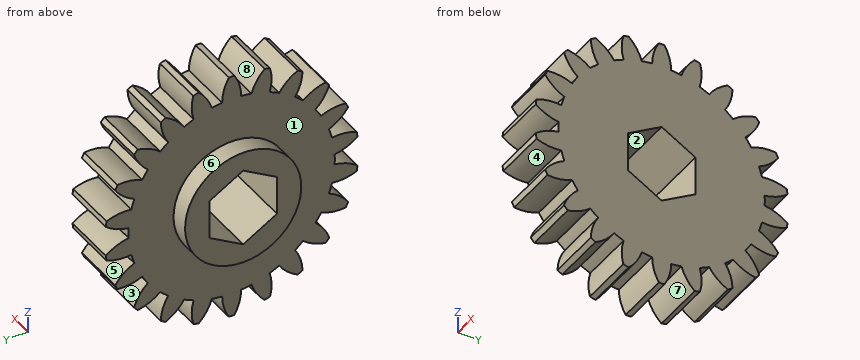
```python
from build123d import *

# Parameters (mm, degrees)
BASPROSKE_W         = 6.604
BASPROSKE_H         = 15.24
TOOTHCUT_DEPTH      = 23.541695056
TEETHCUTS_COUNT     = 22
TEETHCUTS_ANGLE     = 343.636363636
BORSKE_R            = 0.499999
BORE_DEPTH          = 50.8000508
SKETCH1_R           = 6.985
BOSS_EXTRUDE1_DEPTH = 2.286
CUT_EXTRUDE1_DEPTH  = 24.241702632


with BuildPart() as part:
    # BasProSke → Base-Revolve (revolve)
    with BuildSketch(Plane(origin=(0, 0, 0), x_dir=(1, 0, 0), z_dir=(0, 1, 0)), mode=Mode.PRIVATE) as base_revolve_sk:
        with Locations((3.302, 7.62)):
            Rectangle(BASPROSKE_W, BASPROSKE_H)
    revolve(base_revolve_sk.sketch.rotate(Axis((-10, 0, 0), (1, 0, 0)), 180), axis=Axis((-10, 0, 0), (1, 0, 0)))

    # TooCutSke → ToothCut (cut, through all)
    with BuildSketch(Plane(origin=(0, 0, 0), x_dir=(0, 0, -1), z_dir=(1, 0, 0))):
        with BuildLine():
            ThreePointArc((0.629474743, 12.379206137), (0, 12.3952), (-0.629474743, 12.379206137))
            ThreePointArc((-0.629474743, 12.379206137), (-1.05059125, 13.850443254), (-1.855031489, 15.152270303))
            ThreePointArc((-1.855031489, 15.152270303), (0, 15.2654), (1.855031489, 15.152270303))
            ThreePointArc((1.855031489, 15.152270303), (1.05059125, 13.850443254), (0.629474743, 12.379206137))
        make_face()
    toothcut = extrude(amount=TOOTHCUT_DEPTH, mode=Mode.SUBTRACT)

    # TeethCuts: ToothCut ×22 about axis
    teethcuts_axis = Axis((-10, 0, 0), (1, 0, 0))
    for i in range(1, TEETHCUTS_COUNT):
        add(toothcut.rotate(teethcuts_axis, i * TEETHCUTS_ANGLE / (TEETHCUTS_COUNT - 1)), mode=Mode.SUBTRACT)

    # BorSke → Bore (cut, symmetric)
    with BuildSketch(Plane(origin=(0, 0, 0), x_dir=(0, 0, -1), z_dir=(1, 0, 0))):
        with Locations(Location((0, 0, 0), (0, 0, 180))):
            Circle(BORSKE_R)
    extrude(amount=BORE_DEPTH, both=True, mode=Mode.SUBTRACT)

    # Sketch1 → Boss-Extrude1 (add)
    with BuildSketch(Plane.ZY):
        with Locations(Location((0, 0, 0), (0, 0, 180))):
            Circle(SKETCH1_R)
    extrude(amount=BOSS_EXTRUDE1_DEPTH)

    # Sketch2 → Cut-Extrude1 (cut, through all)
    with BuildSketch(Plane(origin=(6.604, 0, 0), x_dir=(0, 0, -1), z_dir=(1, 0, 0))):
        Polygon((2.346351494, 4.064), (-2.346351494, 4.064), (-4.692702988, 0), (-2.346351494, -4.064), (2.346351494, -4.064), (4.692702988, 0), align=None)
    extrude(amount=-CUT_EXTRUDE1_DEPTH, mode=Mode.SUBTRACT)


solid = part.part
```
Part model, mm, in its own coordinate system. Face numbers are marked on the shaded views. A direction names the side the tool comes from. Round coordinates to 2 decimals unless told otherwise and drop trailing zeros. Loops run counter-clockwise (first coordinate to the right, second up) from the corner with the lowest first, then second, coordinate; pieces in that order, holes last.
1. Slice it at B-B (x = -1). Give the cut face in (y, z) (3 decimals), and give its area (3 significant figures).
Solutions:
outline: circle Ø13.97 at (0, 0); hole (-4.064, -2.346) - (0, -4.693) - (4.064, -2.346) - (4.064, 2.346) - (0, 4.693) - (-4.064, 2.346) - close
area: 96.1 mm2
2. Slice it at D-D (z = 3.5). Give the cut face in (x, y).
Solutions:
outline: (-2.29, -6.04) - (0, -6.04) - (0, -11.89) - (6.6, -11.89) - (6.6, -2.07) - (-2.29, -2.07) - close; (-2.29, 2.07) - (6.6, 2.07) - (6.6, 11.89) - (0, 11.89) - (0, 6.04) - (-2.29, 6.04) - close
3. Drill centre lines: line 1 along Z through (x, y) = (5.25, -13); line 2 along Y through (x, z) = (2, -11.5); line 3 along Z through (x, y) = (1, -7). Where is each one in solid material? Low to high.
Solutions:
line 1: z = -6.67 to -4.92, -2.94 to -0.75, 0.75 to 2.94, 4.92 to 6.67
line 2: y = -8.37 to -6.08, -4.63 to 4.63, 6.08 to 8.37
line 3: z = -12.4 to 12.4
4. Slice it at A-A (z = 0). Give the cut face in (x, y) (3 decimals).
Solutions:
outline: (-2.286, -6.985) - (0, -6.985) - (0, -12.395) - (6.604, -12.395) - (6.604, -4.064) - (-2.286, -4.064) - close; (-2.286, 4.064) - (6.604, 4.064) - (6.604, 12.395) - (0, 12.395) - (0, 6.985) - (-2.286, 6.985) - close
5. Slice it at C-C (y = 13). Give the cut face in (x, z), and give its area (3 significant figures).
Solutions:
outline: (0, -6.67) - (6.6, -6.67) - (6.6, -4.92) - (0, -4.92) - close; (0, -2.94) - (6.6, -2.94) - (6.6, -0.75) - (0, -0.75) - close; (0, 0.75) - (6.6, 0.75) - (6.6, 2.94) - (0, 2.94) - close; (0, 4.92) - (6.6, 4.92) - (6.6, 6.67) - (0, 6.67) - close
area: 52.0 mm2
6. Flat gauge pins, fed straight in: pin 1 (2 mm diameter, centred on x = 0.5, y = -8.5, fed in from +Z); pin 2 (5 mm diameter, centred on x = 3, y = -4.5, fed in from +Z); pin 3 (5 mm diameter, centred on x = 4.5, z = 10.5, fed in from -Y). Where does each tip first touch, or does it go through?
Solutions:
pin 1: stops at z = 13
pin 2: stops at z = 14.71
pin 3: stops at y = -11.73
7. 3-axis set-ups, long thin cutter, end or side, ignore diameter. For the marked faces 4, 5, 6, 7 and 8: which of +Z, -Z, +X, -X, +Y, -Y reach the whole face in a straight line?
Solutions:
face 4: +X, -X
face 5: +X, -X, +Y
face 6: -X
face 7: -Z, +X, -X
face 8: +Z, +X, -X
8. Two-plate mould, pull along Y, no slides. Class the marked faces 1, 2 and 3: pulls with the +Y half, pulls with the -Y half, needs draft (parallel to the pull), parting line crosses it, or undercut.
Solutions:
face 1: needs draft
face 2: undercut
face 3: pulls with the +Y half
